Build history of the part. All positions in model axes, mm. Round coordinates to 2 decimals unless told otherwise and drop trailing zeros. Order: outer loops, then holes, each group sorted by start corner. A loop starts at its lowest first (then second) coordinate and runs counter-clockwise, first axis right, second up. Notation, with made-up numbers: (12, 61) - (41, 61) arc R13 cw to (41, 71) - close; hole circle Ø1 at (-1, -39). An arc over 180 degrees is marked (long way). Write each question's results on one line, items separated by ' | '. Start each with the question number.
```python
from build123d import *

# Parameters (mm, degrees)
SKETCH1_W                      = 26
SKETCH1_H                      = 35
BOSS_EXTRUDE1_DEPTH            = 1.5
M3_CLEARANCE_HOLE1_D           = 3.4
M3_CLEARANCE_HOLE1_DEPTH       = 3
M3_CLEARANCE_HOLE1_CSINK_D     = 3.45
M3_CLEARANCE_HOLE1_CSINK_ANGLE = 90
SKETCH4_R                      = 9.5
CUT_EXTRUDE1_DEPTH             = 44.626253564


with BuildPart() as part:
    # Sketch1 → Boss-Extrude1 (new body)
    with BuildSketch(Plane(origin=(0, 0, 0), x_dir=(1, 0, 0), z_dir=(0, 1, 0))):
        with Locations((13, 17.5)):
            Rectangle(SKETCH1_W, SKETCH1_H)
    extrude(amount=BOSS_EXTRUDE1_DEPTH)

    # M3 Clearance Hole1
    with Locations(Plane(origin=(0, 1.5, 0), x_dir=(1, 0, 0), z_dir=(0, 1, 0))):
        with Locations((2.5, 32.5), (2.5, 10.5), (23.5, 10.5), (23.5, 32.5)):
            CounterSinkHole(M3_CLEARANCE_HOLE1_D / 2, M3_CLEARANCE_HOLE1_CSINK_D / 2, depth=M3_CLEARANCE_HOLE1_DEPTH, counter_sink_angle=M3_CLEARANCE_HOLE1_CSINK_ANGLE)

    # Sketch4 → Cut-Extrude1 (cut, through all)
    with BuildSketch(Plane(origin=(0, 1.5, 0), x_dir=(1, 0, 0), z_dir=(0, 1, 0))):
        with Locations(Location((13, 20, 0), (0, 0, 270))):
            Circle(SKETCH4_R)
    extrude(amount=-CUT_EXTRUDE1_DEPTH, mode=Mode.SUBTRACT)


solid = part.part
```
1. Cut at B-B (x = 13). List the corners of the cut face in (y, z).
2. Cut at C-C (z = -20). List the corners of the cut face in (x, y).
3. Cut at A-A (z = -32.5). List the corners of the cut face in (x, y) (3 decimals), plus the area to 3 significant figures.
4. Wall check: line 1 (X direction, y = 0.4, z = -32.5); line 2 (Z direction, x = 23.5, y = 0.9); line 3 (X direction, y = 0.75, z = -31.5). Give the ranges that are in metal, low to high. Write a range as from..to.
5. Mould opens along X. For faces 1 (the face through (22.7, 0.7, -31)), 2 (the face through (13, 0, -10)), 3 (the face through (0, 1, -17)) say: pulls with the +X half, pulls with the -X half, needs draft (parallel to the pull), parting line crosses it, or undercut.
6. Cut at D-D (y = 0.9). List the corners of the cut face in (x, z), plus the area to 3 significant figures.
A:
1) outline: (0, -35) - (1.5, -35) - (1.5, -29.5) - (0, -29.5) - close; (0, -10.5) - (1.5, -10.5) - (1.5, 0) - (0, 0) - close
2) outline: (0, 0) - (3.5, 0) - (3.5, 1.5) - (0, 1.5) - close; (22.5, 0) - (26, 0) - (26, 1.5) - (22.5, 1.5) - close
3) outline: (0, 0) - (0.8, 0) - (0.8, 1.475) - (0.775, 1.5) - (0, 1.5) - close; (4.2, 0) - (21.8, 0) - (21.8, 1.475) - (21.775, 1.5) - (4.225, 1.5) - (4.2, 1.475) - close; (25.2, 0) - (26, 0) - (26, 1.5) - (25.225, 1.5) - (25.2, 1.475) - close | area: 28.8 mm^2
4) line 1: x = 0..0.8, 4.2..21.8, 25.2..26 | line 2: z = -35..-34.2, -30.8..-12.2, -8.8..0 | line 3: x = 0..1.13, 3.87..22.13, 24.87..26
5) face 1: undercut | face 2: needs draft | face 3: pulls with the -X half
6) outline: (0, -35) - (26, -35) - (26, 0) - (0, 0) - close; hole circle Ø3.4 at (2.5, -32.5); hole circle Ø3.4 at (2.5, -10.5); hole circle Ø19 at (13, -20); hole circle Ø3.4 at (23.5, -32.5); hole circle Ø3.4 at (23.5, -10.5) | area: 590 mm^2
